Geometry check sheet. Reference: drawing and pictorial views, mm from the part's lowest x, y, z. Give positions to 0.01 mm unless a question says otherwise; leave off trailing zeros. Order: outer loops, then holes, each group sorted by start corner. A loop starts at its lowest first (then second) coordinate and runs counter-clockwise, first axis right, second up. Notation, with made-up numbers: (69.5, -8) - (121.5, -8) arc R25 ccw to (121.5, 24) - close; hole circle Ø2 at (53, 5). An arc over 180 degrees is marked (long way). Answer in a Markdown table with one row per item.
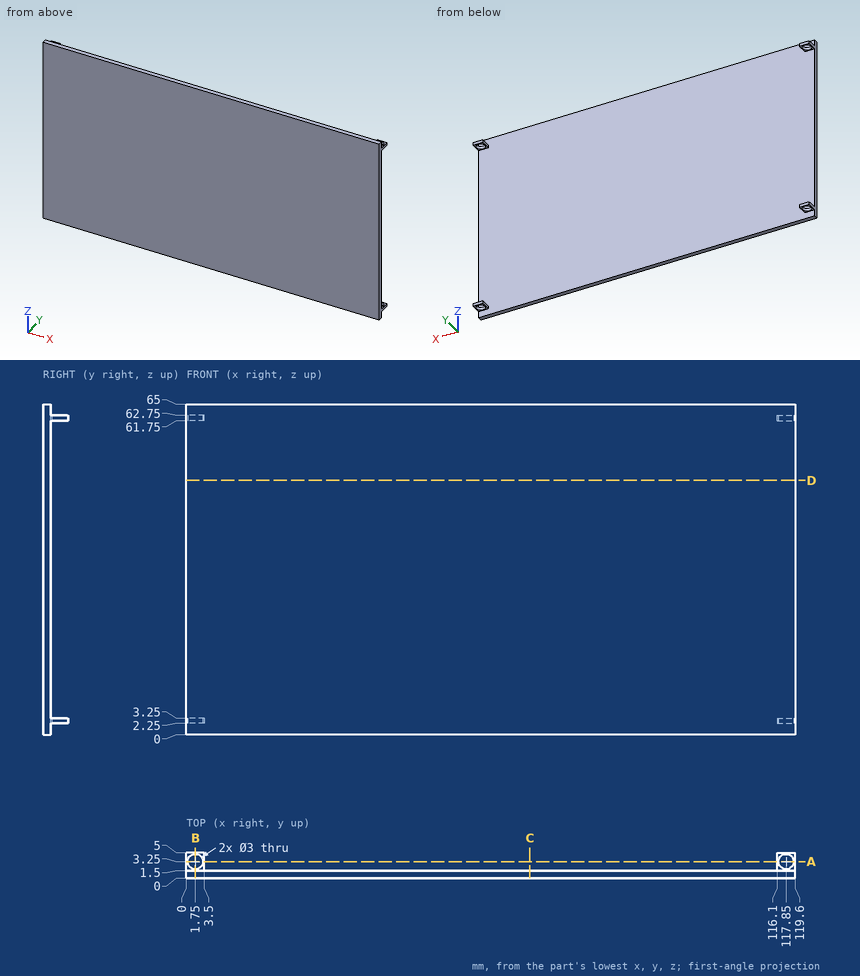
(1) Thickness scan on L1, parallel to X at y = 3.25, z = 2.9; L2, parallel to Y at x = 1.75, z = 2.5; L3, parallel to Y at x = 87, z = 6.5. Record the ranges inside material, lowest first.
Geometry says:
| item | result |
|---|---|
| L1 | 0 to 0.25, 3.25 to 3.5, 116.1 to 116.35, 119.35 to 119.6 |
| L2 | 0 to 1.75, 4.75 to 5 |
| L3 | 0 to 1.5 |
(2) Cross-section at C-C, the plane x = 67.5. Record the cut outline in (y, z), then the cut area to 3 significant figures.
Geometry says:
| item | result |
|---|---|
| outline | (0, 0) - (1.5, 0) - (1.5, 65) - (0, 65) - close |
| area | 97.5 mm² |
(3) Cross-section at B-B, the plane x = 1.75. Record the cut outline in (y, z).
Geometry says:
| item | result |
|---|---|
| outline | (0, 0) - (1.5, 0) - (1.5, 2.25) - (1.75, 2.25) - (1.75, 3.25) - (1.5, 3.25) - (1.5, 61.75) - (1.75, 61.75) - (1.75, 62.75) - (1.5, 62.75) - (1.5, 65) - (0, 65) - close; (4.75, 2.25) - (5, 2.25) - (5, 3.25) - (4.75, 3.25) - close; (4.75, 61.75) - (5, 61.75) - (5, 62.75) - (4.75, 62.75) - close |
(4) Cross-section at A-A, the plane y = 3.25. Give the number of separate pieces and of enclosed holes in the cut face, then the cut area to 3 significant figures.
Geometry says:
| item | result |
|---|---|
| separate pieces | 8 |
| enclosed holes | 0 |
| area | 2.00 mm² |
(5) Cross-section at D-D, the plane z = 50. Record the cut outline in (x, y).
Geometry says:
| item | result |
|---|---|
| outline | (0, 0) - (119.6, 0) - (119.6, 1.5) - (0, 1.5) - close |
(6) Gauge pin test, flat ends, axial feed: P1, Ø1.5, axis at x = 35.5, z = 9, coming from the +Y side; P2, Ø1.8, axis at x = 118, y = 4, coming from the -Z side; P3, Ø3, axis at x = 1.5, y = 3.5, coming from the +Z side. Record the tip position at first contact, or that the pin passes through.
Geometry says:
| item | result |
|---|---|
| P1 | y = 1.5 |
| P2 | z = 2.25 |
| P3 | z = 62.75 |
